```python
from build123d import *

# Parameters (mm, degrees)
SKETCH1_R          = 0.5
BASE_FLANGE1_DEPTH = 0.3


# Sheet-metal steps are written as plain solids
with BuildPart() as part:
    # Sketch1 → Base-Flange1 (new body)
    with BuildSketch(Plane(origin=(0, 0, 0), x_dir=(1, 0, 0), z_dir=(0, 1, 0))):
        with BuildLine():
            Line((-1, 0), (-1, 5))
            ThreePointArc((-1, 5), (0, 6), (1, 5))
            Line((1, 5), (1, 0))
            Line((1, 0), (1.5, 0))
            Line((1.5, 0), (1.5, -1.6))
            Line((1.5, -1.6), (-1.5, -1.6))
            Line((-1.5, -1.6), (-1.5, 0))
            Line((-1.5, 0), (-1, 0))
        make_face()
        with Locations(Location((0, 5, 0), (0, 0, 270))):
            Circle(SKETCH1_R, mode=Mode.SUBTRACT)
    extrude(amount=-BASE_FLANGE1_DEPTH)


solid = part.part
```
Can you work these out from the model? Positions are in its coordinate system, mm. Give positions to 0.01 mm unless a question says otherwise; leave off trailing zeros. Loops run counter-clockwise (first coordinate to the right, second up) from the corner with the lowest first, then second, coordinate; pieces in that order, holes last. Notation, with made-up numbers: M 69.5,23.25 L 118.5,23.25 A12 ccw 118.5,46.25 Z; hole C -26.75,-4 d10. An arc over 180 degrees is marked long. Use CSV: the item, a comma, the result in double quotes. Start each with the question number.
1. For P1, Ø1.5, axis at x = 0.5, z = -5, coming from the +Y side, with a flat end and sliding along its axis, tell me the tip position at first contact or that it passes through.
2. Imagine slicing it at B-B, the plane y = -0.2. Write out the boundary of the cut face in (x, z).
3. If I drill on L1, parallel to X at y = -0.1, z = -5; L2, parallel to Z at x = -0.05, y = -0.15; L3, parallel to Z at x = 1.2, y = -0.1, over which ranges is the centre line in solid material (lowest first)?
4. Imagine slicing it at C-C, the plane z = -3.5. Write out the boundary of the cut face in (x, y).
5. If we mould it in two halves opening along X, with no side actions, what happens to faces 1 (the face through (0, 0, -1)), 2 (the face through (-0.02, -0.15, -6))? For each: released by +X, released by -X, zero draft, split by the parting line, or undercut.
6. Imagine slicing it at A-A, the plane x = 0. Write out the boundary of the cut face in (y, z).
Response values:
1,P1,"y = 0"
2,outline,"M -1.5,0 L -1,0 L -1,-5 A1 ccw 1,-5 L 1,0 L 1.5,0 L 1.5,1.6 L -1.5,1.6 Z; hole C 0,-5 d1"
3,L1,"-1 to -0.5, 0.5 to 1"
3,L2,"-6 to -5.5, -4.5 to 1.6"
3,L3,"0 to 1.6"
4,outline,"M -1,-0.3 L 1,-0.3 L 1,0 L -1,0 Z"
5,face 1,"zero draft"
5,face 2,"split by the parting line"
6,outline,"M -0.3,-6 L 0,-6 L 0,-5.5 L -0.3,-5.5 Z; M -0.3,-4.5 L 0,-4.5 L 0,1.6 L -0.3,1.6 Z"
